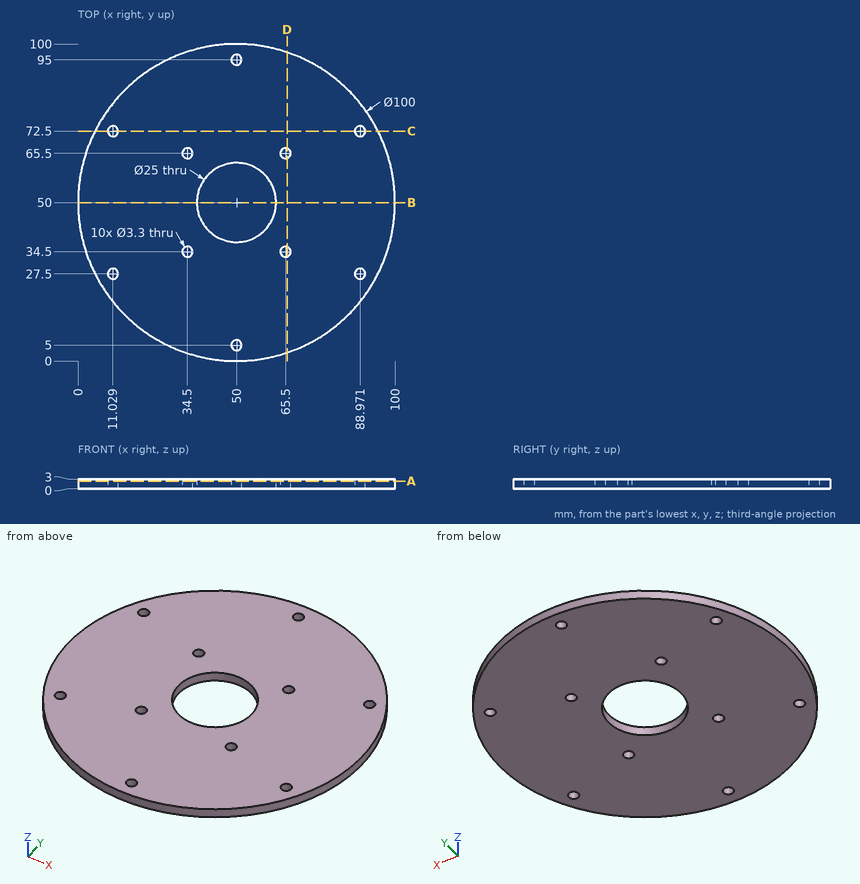
Check sheet for the drawn part. Datum: minimum x, y, z corner. Units: mm. Give positions to 0.01 mm unless a question says otherwise; leave off trailing zeros. Loops run counter-clockwise (first coordinate to the right, second up) from the corner with the lowest first, then second, coordinate; pieces in that order, holes last.
1) Sectioned sample at B-B, the plane y = 50. Enter the section's corners in (x, z), then the cut area to 3 significant figures.
2) Sectioned sample at D-D, the plane x = 66. Enter the section's corners in (y, z).
3) Depth check by flat-ended pin: pin 1 Ø1 at (y, z) = (37.5, 2.5) entering from -X. Enter the tip coordinate at first touch or a pass-through.
4) Sectioned sample at C-C, the plane y = 72.5. Enter the section's corners in (x, z).
5) Thickness scan on line 1 along X through (y, z) = (28, 1.5); line 2 along Y through (x, z) = (50, 0.9); line 3 along X through (y, z) = (65.5, 1). Record the ranges inside material, lowest first.
6) Sectioned sample at A-A, the plane z = 2.3. Count the separate pieces of the cut face and the enclosed holes in it, then the cut area to 3 significant figures.
Answers:
1. outline: (0, 0) - (37.5, 0) - (37.5, 3) - (0, 3) - close; (62.5, 0) - (100, 0) - (100, 3) - (62.5, 3) - close
1. area: 225 mm2
2. outline: (2.63, 0) - (32.93, 0) - (32.93, 3) - (2.63, 3) - close; (36.07, 0) - (63.93, 0) - (63.93, 3) - (36.07, 3) - close; (67.07, 0) - (97.37, 0) - (97.37, 3) - (67.07, 3) - close
3. pin 1: stops at x = 1.46
4. outline: (5.35, 0) - (9.38, 0) - (9.38, 3) - (5.35, 3) - close; (12.68, 0) - (87.32, 0) - (87.32, 3) - (12.68, 3) - close; (90.62, 0) - (94.65, 0) - (94.65, 3) - (90.62, 3) - close
5. line 1: x = 5.1 to 9.46, 12.6 to 87.4, 90.54 to 94.9
5. line 2: y = 0 to 3.35, 6.65 to 37.5, 62.5 to 93.35, 96.65 to 100
5. line 3: x = 2.46 to 32.85, 36.15 to 63.85, 67.15 to 97.54
6. separate pieces: 1
6. enclosed holes: 11
6. area: 7,280 mm2
